The listing builds one solid part. Answer for the finished solid, in the listing's coordinates (mm). A direction names the side the tool comes from. Round coordinates to 2 decimals unless told otherwise and drop trailing zeros. Write each loop counter-clockwise with the first axis right and the second up, starting at its lowest first coordinate (ties: lowest second). Pieces come first, ordered by that corner, then holes. Notation, with made-up numbers: M 5,34 L 49,34 A12 ccw 49,40 Z; hole C 30,-22.75 d9. An arc over 180 degrees is marked long. One line per item, written item: value. Start each with the question number.
(1) For a pull along Y with two mould halves and no side action, classify faces 1 (the cylindrical face through (1.85, -10.07, 17.73)), 2 (the flat face through (0, 0, 6)) as released by +Y, released by -Y, zero draft, split by the parting line, or undercut.
(2) For faces 3 (the flat face through (3.761, 0, -6)), 4 (the cylindrical face through (1.854, -3.215, 5.476)), determine the directions among +Z, -Z, +X, -X, +Y, -Y from which every point of the face is accessible in a straight line to the end or side of a thin tool.
(3) Section A-A (x = 2.95) is taken. Determine the outline of the cut face in (y, z) (3 decimals).
(4) Section B-B (z = 8) is taken. State how many separate pieces and enclosed holes the cut face has, plus the area to 3 significant figures.
(5) Given P1, Ø1, axis at x = 2, y = 1, coming from the +Z side; P2, Ø1.5, axis at x = 3, z = 20.5, coming from the -Y side; P3, Ø2, axis at x = 2.5, y = -15.5, coming from the -Z side; P4, Ø2.5, axis at y = 0, z = 0, coming from the +X side, each flat-ended and moving along its own axis, determine where each tip first touches the part or whether it passes through.
(6) Consider probe 1 along Y at (x, z) = (2.05, 5.5); probe 2 along Z at (x, y) = (2.6, -8.5); probe 3 along Y at (x, z) = (1.3, -8). Determine where each line is inside the solid, lowest interval first.
```python
from build123d import *

# Parameters (mm, degrees)
F3_DEPTH      = 82
F3_DEPTH_BACK = 25.4
F4_R          = 1.6002
F5_DEPTH      = 3.7619021022


# Not quite as in the source:
# - an extrude ends at something that could not be found from the text; its depth is read off the source's solid


with BuildPart() as f1:
    # F0 (on Front) → F1 (revolve)
    with BuildSketch(Plane.XZ):
        with BuildLine():
            Line((0, 28.125), (0, 0))
            Line((0, 0), (3.7609021022, 0))
            Line((3.7609021022, 0), (3.7609021022, 28.125))
            ThreePointArc((3.7609021022, 28.125), (1.8804510511, 27.2531215698), (0, 28.125))
        make_face()
    revolve(axis=Axis((1.8804510511, 0, 0), (1, 0, 0)))

    # F2 (on Right) → F3 (cut, two sides)
    with BuildSketch(Plane.YZ) as f3_sk:
        with BuildLine():
            ThreePointArc((-5.499261314, 3.175), (-3.175, 5.499261314), (0, 6.35))
            Line((0, 6.35), (0, 20.391961195))
            ThreePointArc((0, 20.391961195), (-10.1959805975, 17.6599564279), (-17.6599564279, 10.1959805975))
            Line((-17.6599564279, 10.1959805975), (-5.499261314, 3.175))
        make_face()
        with BuildLine():
            Line((0, -20.391961195), (0, -6.35))
            ThreePointArc((0, -6.35), (-3.175, -5.499261314), (-5.499261314, -3.175))
            Line((-5.499261314, -3.175), (-17.6599564279, -10.1959805975))
            ThreePointArc((-17.6599564279, -10.1959805975), (-10.1959805975, -17.6599564279), (0, -20.391961195))
        make_face()
        with BuildLine():
            ThreePointArc((5.499261314, 3.175), (6.1336289969, 1.6435009364), (6.35, 0))
            ThreePointArc((6.35, 0), (6.1336289969, -1.6435009364), (5.499261314, -3.175))
            Line((5.499261314, -3.175), (17.6599564279, -10.1959805975))
            ThreePointArc((17.6599564279, -10.1959805975), (19.6971219669, -5.2778279243), (20.391961195, 0))
            ThreePointArc((20.391961195, 0), (19.6971219669, 5.2778279243), (17.6599564279, 10.1959805975))
            Line((17.6599564279, 10.1959805975), (5.499261314, 3.175))
        make_face()
    extrude(amount=-F3_DEPTH, mode=Mode.SUBTRACT)
    extrude(f3_sk.sketch, amount=F3_DEPTH_BACK, mode=Mode.SUBTRACT)

    # F4 (on face) → F5 (cut, through all)
    with BuildSketch(Plane(origin=(0, 0, 0), x_dir=(0, -1, 0), z_dir=(-1, 0, 0))):
        Circle(F4_R)
    extrude(amount=-F5_DEPTH, mode=Mode.SUBTRACT)


solid = f1.part
```
Recorded:
1. face 1: undercut
1. face 2: zero draft
2. face 3: +Z, -Z, +X, +Y, -Y
2. face 4: +X, -X
3. outline: C 0,0 d54.995; hole M -17.66,-10.196 A20.392 ccw 0,-20.392 L 0,-6.35 A6.35 cw -5.499,-3.175 Z; hole M -17.66,10.196 L -5.499,3.175 A6.35 cw 0,6.35 L 0,20.392 A20.392 ccw Z; hole C 0,0 d3.2; hole M 5.499,-3.175 L 17.66,-10.196 A20.392 ccw 17.66,10.196 L 5.499,3.175 A6.35 cw Z
4. separate pieces: 3
4. enclosed holes: 0
4. area: 128 mm2
5. P1: stops at z = 27.32
5. P2: stops at y = -19.48
5. P3: stops at z = -23.36
5. P4: passes through
6. probe 1: y = -26.7 to -9.53, -3.17 to 9.53, 19.64 to 26.7
6. probe 2: z = -26.01 to -18.54, -4.91 to 4.91, 18.54 to 26.01
6. probe 3: y = -26.13 to -13.86, 0 to 13.86, 18.76 to 26.13
